Read the model definition and answer for the solid it produces. Units are mm, in the model's axes. Face numbers are marked on the shaded views. A direction names the side the tool comes from. Round coordinates to 2 decimals unless told otherwise and drop trailing zeros. Write each loop counter-clockwise with the first axis right and the second up, starting at its lowest first coordinate (ties: lowest second). Pieces come first, ordered by that corner, then holes. Notation, with made-up numbers: (-36, -35) - (-16, -35) arc R34 cw to (-16, 2) - close; hole circle Ø1 at (47, 40). An arc over 180 degrees is marked (long way). One line per item, written item: value. Start each with the question number.
(1) A cutting plane is placed at D-D, the plane x = 0. Determine the outline of the cut face in (y, z), plus the area to 3 significant figures.
(2) A cutting plane is placed at C-C, the plane y = -6. Determine the outline of the cut face in (x, z), plus the area to 3 significant figures.
(3) Flat-ended cylindrical pins translate along their axes: pin 1 Ø1.5 at (y, z) = (-7.5, 10) entering from +X; pin 2 Ø6 at (x, y) = (20, -8.5) entering from -Z; pin 3 Ø5 at (x, y) = (32.5, -9) entering from +Z. Find the tip coordinate at first contact, or state that the pin passes through.
(4) The mould has two halves that part along Z. Classify the marked faces 4, 5 and 6: +Z half, -Z half, draft (parallel to the pull), parting line (faces both ways), or undercut.
(5) For the marked faces 1, 2 and 3, determine the directions among +Z, -Z, +X, -X, +Y, -Y from which every point of the face is accessible in a straight line to the end or side of a thin tool.
(6) A cutting plane is placed at A-A, the plane x = 85. Determine the outline of the cut face in (y, z).
(7) Find the intervals of material crossed by L1, parallel to Z at x = 85, y = -15; L2, parallel to Z at x = 24, y = -1; L3, parallel to Y at x = 11, z = 4.75, in increasing order.
(8) A cutting plane is placed at B-B, the plane z = -3.5. Determine the outline of the cut face in (x, y).
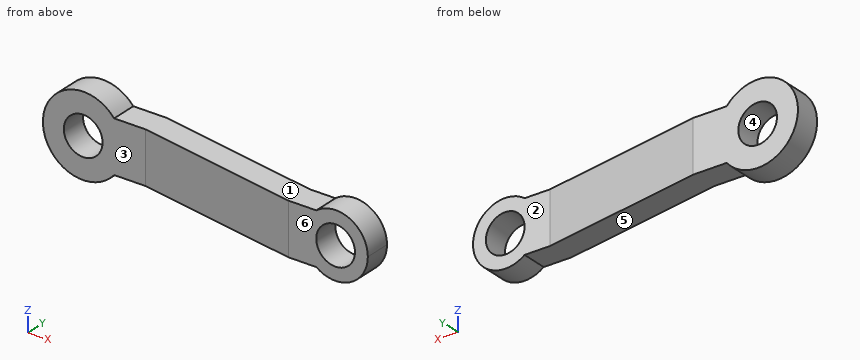
from build123d import *

# Parameters (mm, degrees)
F0_R     = 6
F1_DEPTH = 25
F3_DEPTH = 12.5


with BuildPart() as f1:
    # F0 (on Front) → F1 (new body)
    with BuildSketch(Plane.XZ):
        with BuildLine():
            ThreePointArc((9.604686, -8), (11.753905, -4.253905), (12.5, 0))
            ThreePointArc((12.5, 0), (11.753905, 4.253905), (9.604686, 8))
            ThreePointArc((9.604686, 8), (-12.5, 0), (9.604686, -8))
        make_face()
        Circle(F0_R, mode=Mode.SUBTRACT)
        with BuildLine():
            ThreePointArc((95, 0), (89.472136, 8.944272), (79, 8))
            ThreePointArc((79, 8), (75, 0), (79, -8))
            ThreePointArc((79, -8), (89.472136, -8.944272), (95, 0))
        make_face()
        with Locations((85, 0)):
            Circle(F0_R, mode=Mode.SUBTRACT)
        with BuildLine():
            ThreePointArc((9.604686, 8), (11.753905, 4.253905), (12.5, 0))
            ThreePointArc((12.5, 0), (11.753905, -4.253905), (9.604686, -8))
            Line((9.604686, -8), (79, -8))
            ThreePointArc((79, -8), (75, 0), (79, 8))
            Line((79, 8), (9.604686, 8))
        make_face()
    extrude(amount=F1_DEPTH)

    # F2 (on Top) → F3 (intersect, symmetric)
    with BuildSketch(Plane.XY):
        Polygon((20, 0), (-12.5, 0), (-12.5, -8), (19.300091, -8), (70.341627, -17), (95, -17), (95, -9), (71.041536, -9), align=None)
    extrude(amount=F3_DEPTH, both=True, mode=Mode.INTERSECT)


solid = f1.part
Here are the results:
1. outline: (-8, -12.5) - (0, -12.5) - (0, -6) - (-8, -6) - close; (-8, 6) - (0, 6) - (0, 12.5) - (-8, 12.5) - close
1. area: 104 mm²
2. outline: (9.6, -8) - (54.03, -8) - (54.03, 8) - (9.6, 8) arc R12.5 ccw (long way) to start; hole circle Ø12 at (0, 0)
2. area: 1,060 mm²
3. pin 1: x = 8.41
3. pin 2: z = -8
3. pin 3: z = 8
4. face 4: undercut
4. face 5: -Z half
4. face 6: draft
5. face 1: +Z, +Y, -Y
5. face 2: +Z, -Z, +X, +Y
5. face 3: +Z, -Z, -X, -Y
6. outline: (-17, -10) - (-9, -10) - (-9, -6) - (-17, -6) - close; (-17, 6) - (-9, 6) - (-9, 10) - (-17, 10) - close
7. L1: -10 to -6, 6 to 10
7. L2: -8 to 8
7. L3: -8 to 0
8. outline: (-12, -8) - (-4.87, -8) - (-4.87, 0) - (-12, 0) - close; (4.87, -8) - (19.3, -8) - (70.34, -17) - (80.13, -17) - (80.13, -9) - (71.04, -9) - (20, 0) - (4.87, 0) - close; (89.87, -17) - (94.37, -17) - (94.37, -9) - (89.87, -9) - close
